from build123d import *

# Parameters (mm, degrees)
SKETCH1_W           = 33.528
SKETCH1_H           = 33.528
BOSS_EXTRUDE1_DEPTH = 3.175
SKETCH2_W           = 19.05
SKETCH2_H           = 19.05
CUT_EXTRUDE1_DEPTH  = 3.175
SKETCH3_R           = 1.778
CUT_EXTRUDE2_DEPTH  = 3.175


with BuildPart() as part:
    # Sketch1 → Boss-Extrude1 (new body)
    with BuildSketch(Plane.XY):
        with Locations((16.764, 16.764)):
            Rectangle(SKETCH1_W, SKETCH1_H)
    extrude(amount=BOSS_EXTRUDE1_DEPTH)

    # Sketch2 → Cut-Extrude1 (cut)
    with BuildSketch(Plane.XY.offset(3.175)):
        with Locations((16.764, 16.764)):
            Rectangle(SKETCH2_W, SKETCH2_H)
    extrude(amount=-CUT_EXTRUDE1_DEPTH, mode=Mode.SUBTRACT)

    # Sketch3 → Cut-Extrude2 (cut)
    with BuildSketch(Plane.XY.offset(3.175)):
        with Locations((30.2387, 30.2387)):
            Circle(SKETCH3_R)
        with Locations((30.2387, 3.2893)):
            Circle(SKETCH3_R)
        with Locations(Location((3.2893, 3.2893, 0), (0, 0, 180))):
            Circle(SKETCH3_R)
        with Locations(Location((3.2893, 30.2387, 0), (0, 0, 180))):
            Circle(SKETCH3_R)
    extrude(amount=-CUT_EXTRUDE2_DEPTH, mode=Mode.SUBTRACT)


solid = part.part
Design review of the part built by this model. Coordinates are the model's own, in mm. A direction names the side the tool comes from. Coordinates: 2 decimals unless noted, no trailing zeros. Order: outer loops, then holes, each group sorted by start corner. A loop starts at its lowest first (then second) coordinate and runs counter-clockwise, first axis right, second up. Notation, with made-up numbers: (14.5, 15) -> (63.5, 15) arc R28 cw to (63.5, 34) -> close; hole circle Ø8 at (-2, -25). An arc over 180 degrees is marked (long way). One line per item, written item: value.
1) We need section C-C, the plane z = 1.35. Give the boundary of the cut face in (x, y).
Output values:
outline: (0, 0) -> (33.53, 0) -> (33.53, 33.53) -> (0, 33.53) -> close; hole circle Ø3.56 at (3.29, 3.29); hole circle Ø3.56 at (3.29, 30.24); hole (7.24, 7.24) -> (26.29, 7.24) -> (26.29, 26.29) -> (7.24, 26.29) -> close; hole circle Ø3.56 at (30.24, 3.29); hole circle Ø3.56 at (30.24, 30.24)
2) Draft analysis for pull direction X (two halves, no side actions). For faces 3 (the face through (5, 17, 0)), 4 (the face through (17, 7.239, 2)), 5 (the face through (0, 17, 2)), state which applies: +X half, -X half, draft (parallel to the pull), parting line (faces both ways), or undercut.
Output values:
face 3: draft
face 4: undercut
face 5: -X half
3) We need section D-D, the plane y = 2.5. Give the boundary of the cut face in (x, z) (1 decimal), then the cut area to 3 significant figures.
Output values:
outline: (0, 0) -> (1.7, 0) -> (1.7, 3.2) -> (0, 3.2) -> close; (4.9, 0) -> (28.6, 0) -> (28.6, 3.2) -> (4.9, 3.2) -> close; (31.8, 0) -> (33.5, 0) -> (33.5, 3.2) -> (31.8, 3.2) -> close
area: 86.2 mm2
4) Machinability: for faces 1 (the face through (26.289, 17, 2)), 2 (the face through (33.528, 17, 2)), which of the approach directions +Z, -Z, +X, -X, +Y, -Y give a long, thin tool a straight path to every point of the face, cutting with its end or side? Answer none if there is none.
Output values:
face 1: +Z, -Z
face 2: +Z, -Z, +X, +Y, -Y
5) To check wall thickness, follow probe 1 along X at (y, z) = (25, 0.9); probe 2 along Y at (x, z) = (4.5, 2.4). State the ranges of each line that lie inside material, in increasing order. Write a range as [from, to].
Output values:
probe 1: x = [0, 7.24], [26.29, 33.53]
probe 2: y = [0, 1.99], [4.59, 28.94], [31.54, 33.53]
6) We need section A-A, the plane y = 24. Give the boundary of the cut face in (x, z) (3 decimals).
Output values:
outline: (0, 0) -> (7.239, 0) -> (7.239, 3.175) -> (0, 3.175) -> close; (26.289, 0) -> (33.528, 0) -> (33.528, 3.175) -> (26.289, 3.175) -> close
